from build123d import *

# Parameters (mm, degrees)
SKETCH1_W               = 12.7
SKETCH1_H               = 12.7
BOSS_EXTRUDE1_DEPTH     = 34.925
F_1_4_20_TAPPED_HOLE1_D = 6.35
F_1_4_20_TAPPED_HOLE2_D = 6.35
SKETCH6_W               = 12.7
SKETCH6_H               = 39.6875
SKETCH6_R               = 3.175
CUT_EXTRUDE1_DEPTH      = 13.7


with BuildPart() as part:
    # Sketch1 → Boss-Extrude1 (new body, symmetric)
    with BuildSketch(Plane.XY):
        Rectangle(SKETCH1_W, SKETCH1_H)
    extrude(amount=BOSS_EXTRUDE1_DEPTH, both=True)

    # 1/4-20 Tapped Hole1 (through all)
    with Locations(Plane(origin=(0, 6.35, 0), x_dir=(1, 0, 0), z_dir=(0, 1, 0))):
        with Locations((0, 0), (0, 19.05), (0, -19.05)):
            Hole(F_1_4_20_TAPPED_HOLE1_D / 2)

    # 1/4-20 Tapped Hole2 (through all)
    with Locations(Plane(origin=(6.35, 0, 0), x_dir=(0, 0, -1), z_dir=(1, 0, 0))):
        with Locations((9.525, 0), (28.575, 0), (-9.525, 0), (-28.575, 0)):
            Hole(F_1_4_20_TAPPED_HOLE2_D / 2)

    # Sketch6 → Cut-Extrude1 (cut, through all)
    with BuildSketch(Plane(origin=(0, 6.35, 0), x_dir=(1, 0, 0), z_dir=(0, 1, 0))):
        with Locations((0, 15.08125)):
            Rectangle(SKETCH6_W, SKETCH6_H)
        Circle(SKETCH6_R, mode=Mode.SUBTRACT)
        with Locations((0, 19.05)):
            Circle(SKETCH6_R, mode=Mode.SUBTRACT)
    extrude(amount=-CUT_EXTRUDE1_DEPTH, mode=Mode.SUBTRACT)


solid = part.part
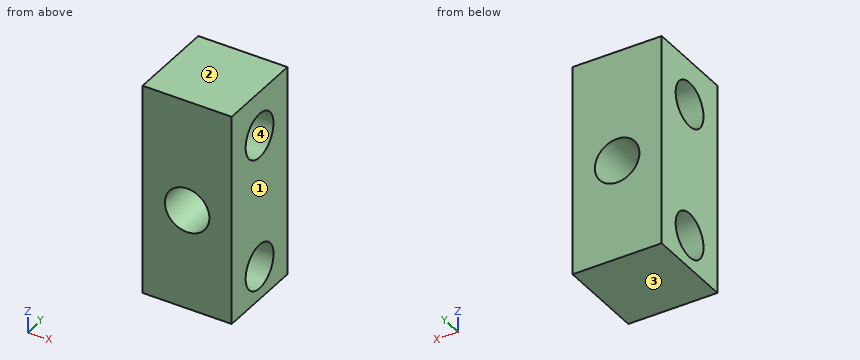
Geometry check sheet. Reference: the model listing, model coordinates, mm. Face numbers are marked on the shaded views. Give positions to 0.01 mm unless a question says otherwise; leave off trailing zeros. Loops run counter-clockwise (first coordinate to the right, second up) from the corner with the lowest first, then second, coordinate; pieces in that order, holes last. Notation, with made-up numbers: (-24, 64.25) -> (-13, 64.25) arc R15 cw to (-13, 85.25) -> close; hole circle Ø3 at (89, 1.5). An arc over 180 degrees is marked (long way). Answer in a Markdown table with one row per item. Add a question column.
1) Cross-section at B-B on z = 19.05. Record the boundary of the cut face in (x, y) (3 decimals), and give its area (3 significant figures).
2) Draft check along Z on the marked faces 1, 2, 3 and 4. Enter one of: pulls with the +Z half, pulls with the -Z half, needs draft (parallel to the pull), parting line crosses it, or undercut.
3) Gauge pin test, flat end, axial feed: P1, Ø5, axis at y = 0, z = 9.525, coming from the -X side. Record the tip position at first contact, or that the pin passes through.
4) Cross-section at A-A on x = 0. State how many separate pieces and enclosed holes the cut face has, and give its area (3 significant figures).
5) Material ranges on probe 1 along Z at (x, y) = (1, -0.5) (1 decimal); probe 2 along Z at (x, y) = (5, 0.5) (1 decimal); probe 3 along Z at (x, y) = (-5.5, 1.75) (1 decimal), recorded low to high. Write a range as from..to.
Outcome:
| question | item | result |
|---|---|---|
| 1 | outline | (-6.35, -6.35) -> (-3.175, -6.35) -> (-3.175, 6.35) -> (-6.35, 6.35) -> close; (3.175, -6.35) -> (6.35, -6.35) -> (6.35, 6.35) -> (3.175, 6.35) -> close |
| 1 | area | 80.6 mm^2 |
| 2 | face 1 | needs draft |
| 2 | face 2 | pulls with the +Z half |
| 2 | face 3 | pulls with the -Z half |
| 2 | face 4 | undercut |
| 3 | P1 | passes through |
| 4 | separate pieces | 2 |
| 4 | enclosed holes | 2 |
| 4 | area | 239 mm^2 |
| 5 | probe 1 | z = 4.8..6.4, 12.7..16, 22.1..25.4, 31.7..34.9 |
| 5 | probe 2 | z = 4.8..6.4, 12.7..25.4, 31.7..34.9 |
| 5 | probe 3 | z = 4.8..6.9, 12.2..25.9, 31.2..34.9 |
